```python
from build123d import *

# Parameters (mm, degrees)
BOSS_EXTRUDE1_DEPTH = 6.35
SKETCH2_W           = 3.302
SKETCH2_H           = 31.75
CUT_EXTRUDE1_DEPTH  = 7.35
SKETCH3_R           = 3.175
CUT_EXTRUDE2_DEPTH  = 7.35
FILLET1_R           = 12.7


with BuildPart() as part:
    # Sketch1 → Boss-Extrude1 (new body)
    with BuildSketch(Plane(origin=(0, 0, 0), x_dir=(1, 0, 0), z_dir=(0, 1, 0))):
        Polygon((-31.75, 0), (31.75, 0), (31.75, 200.66), (82.55, 295.91), (-82.55, 295.91), (-31.75, 200.66), align=None)
    extrude(amount=BOSS_EXTRUDE1_DEPTH)

    # Sketch2 → Cut-Extrude1 (cut, through all)
    with BuildSketch(Plane(origin=(0, 6.35, 0), x_dir=(1, 0, 0), z_dir=(0, 1, 0))):
        with Locations((-17.78, 39.37)):
            Rectangle(SKETCH2_W, SKETCH2_H)
        with Locations((-17.78, 113.03)):
            Rectangle(SKETCH2_W, SKETCH2_H)
        with Locations((-17.78, 186.69)):
            Rectangle(SKETCH2_W, SKETCH2_H)
        with Locations((17.78, 39.37)):
            Rectangle(SKETCH2_W, SKETCH2_H)
        with Locations((17.78, 113.03)):
            Rectangle(SKETCH2_W, SKETCH2_H)
        with Locations((17.78, 186.69)):
            Rectangle(SKETCH2_W, SKETCH2_H)
    extrude(amount=-CUT_EXTRUDE1_DEPTH, mode=Mode.SUBTRACT)

    # Sketch3 → Cut-Extrude2 (cut, through all)
    with BuildSketch(Plane(origin=(0, 6.35, 0), x_dir=(1, 0, 0), z_dir=(0, 1, 0))):
        with Locations((-22.5425, 155.575)):
            Circle(SKETCH3_R)
        with Locations((-22.5425, 142.875)):
            Circle(SKETCH3_R)
        with Locations((22.5425, 142.875)):
            Circle(SKETCH3_R)
        with Locations((22.5425, 155.575)):
            Circle(SKETCH3_R)
        with Locations((-22.479, 9.525)):
            Circle(SKETCH3_R)
        with Locations((22.479, 9.525)):
            Circle(SKETCH3_R)
        with Locations((-22.5425, 82.55)):
            Circle(SKETCH3_R)
        with Locations((-22.5425, 69.85)):
            Circle(SKETCH3_R)
        with Locations((22.5425, 69.85)):
            Circle(SKETCH3_R)
        with Locations((22.5425, 82.55)):
            Circle(SKETCH3_R)
    extrude(amount=-CUT_EXTRUDE2_DEPTH, mode=Mode.SUBTRACT)

    # Fillet1
    fillet1_edges = [part.edges().sort_by_distance(p)[0] for p in [
        (-82.55, 3.175, -295.91),
        (82.55, 3.175, -295.91),
    ]]
    fillet(fillet1_edges, radius=FILLET1_R)


solid = part.part
```
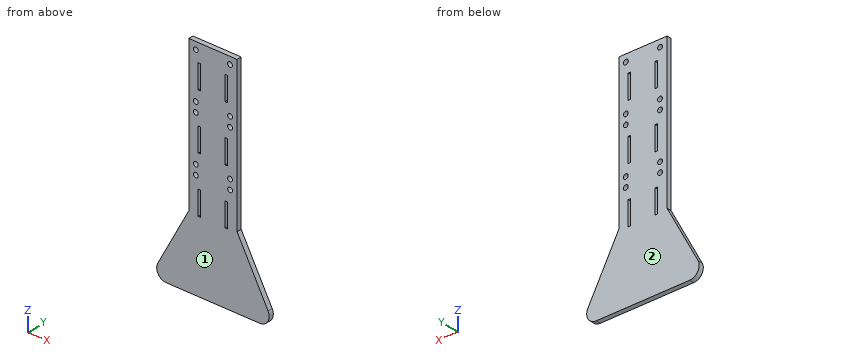
Model file for the job. Use its own axes, mm. Face numbers are marked on the shaded views. Coordinates: 2 decimals unless noted, no trailing zeros. Order: outer loops, then holes, each group sorted by start corner. A loop starts at its lowest first (then second) coordinate and runs counter-clockwise, first axis right, second up. Notation, with made-up numbers: (-5, 84.5) -> (13, 84.5) arc R18 cw to (13, 88.5) -> close; hole circle Ø9 at (-32.5, 21). An arc over 180 degrees is marked (long way). Return JSON: item names as keys, results as strings.
Item 1: Slice it at B-B (x = -48). Write the cut outline in (y, z).
Model answer:
{"outline": "(0, -295.91) -> (6.35, -295.91) -> (6.35, -231.13) -> (0, -231.13) -> close"}
Item 2: Pin check, flat tips, straight feed: P1, Ø3, axis at y = 2, z = -42, coming from the -X side; P2, Ø5, axis at x = 22.479, z = -9.525, coming from the -Y side; P3, Ø3, axis at y = 4, z = -111.5, coming from the +X side; P4, Ø3, axis at x = -42, y = 3, coming from the +Z side. Stop position of each tip, or through.
Model answer:
{"P1": "stops at x = -31.75", "P2": "passes through", "P3": "stops at x = 31.75", "P4": "stops at z = -217.07"}
Item 3: Wall check: line 1 along X through (y, z) = (2.75, -45.5); line 2 along X through (y, z) = (3.75, -82.55); line 3 along Z through (x, y) = (-25, 2). Give the ranges that are in metal, low to high. Write a range as from..to.
Model answer:
{"line 1": "x = -31.75..-19.43, -16.13..16.13, 19.43..31.75", "line 2": "x = -31.75..-25.72, -19.37..19.37, 25.72..31.75", "line 3": "z = -295.91..-157.59, -153.56..-144.89, -140.86..-84.56, -80.54..-71.86, -67.84..-11.46, -7.59..0"}
Item 4: Slice it at D-D (y = 5.25). Count the separate pieces of the cut face and the enclosed holes in it, then the cut area to 3 significant figures.
Model answer:
{"separate pieces": "1", "enclosed holes": "16", "area": "22,500 mm²"}
Item 5: Mould opens along Y. For the marked faces 1 and 2 say: pulls with the +Y half, pulls with the -Y half, needs draft (parallel to the pull), parting line crosses it, or undercut.
Model answer:
{"face 1": "pulls with the -Y half", "face 2": "pulls with the +Y half"}
Item 6: Slice it at C-C (z = -168). Write the cut outline in (x, y).
Model answer:
{"outline": "(-31.75, 0) -> (31.75, 0) -> (31.75, 6.35) -> (-31.75, 6.35) -> close"}
Item 7: Slice it at A-A (z = -82.55). Write the cut outline in (x, y).
Model answer:
{"outline": "(-31.75, 0) -> (-25.72, 0) -> (-25.72, 6.35) -> (-31.75, 6.35) -> close; (-19.37, 0) -> (19.37, 0) -> (19.37, 6.35) -> (-19.37, 6.35) -> close; (25.72, 0) -> (31.75, 0) -> (31.75, 6.35) -> (25.72, 6.35) -> close"}
